The model under review builds one solid part; all positions refer to its coordinate system, in mm. A direction names the side the tool comes from. Round coordinates to 2 decimals unless told otherwise and drop trailing zeros. Loops run counter-clockwise (first coordinate to the right, second up) from the corner with the lowest first, then second, coordinate; pieces in that order, holes last. Notation, with made-up numbers: M 1,-3 L 22,-3 A11 cw 22,2 Z; hole C -24.75,82 d9. An arc over 180 degrees is marked long. Use a Markdown table: item, result. Add a question column.
```python
from build123d import *

# Parameters (mm, degrees)
F2_DEPTH = 381
F0_W     = 914.4
F0_H     = 609.6
F3_DEPTH = 19.05
F4_REACH = 1907.1780931


with BuildPart() as f2:
    # F1 (on Right) → F2 (new body, symmetric)
    with BuildSketch(Plane.YZ):
        Polygon((-197.9734073051, 940.2559094878), (-223.3734073051, 984.25), (-239.8711912472, 974.725), (-204.9461912472, 914.2331255457), (207.4984073051, 1152.3581255457), (197.9734073051, 1168.8559094878), align=None)
    extrude(amount=F2_DEPTH, both=True)



with BuildPart() as f3:
    # F0 (on Top) → F3 (new body)
    with BuildSketch(Plane.XY):
        Rectangle(F0_W, F0_H)
        Polygon((-342.9, -111.5645430735), (-190.5, 152.4), (190.5, 152.4), (342.9, -111.5645430735), (326.4022160579, -121.0895430735), (179.5014773719, 133.35), (-179.5014773719, 133.35), (-326.4022160579, -121.0895430735), align=None, mode=Mode.SUBTRACT)
        Polygon((190.5, 152.4), (-190.5, 152.4), (-342.9, -111.5645430735), (-326.4022160579, -121.0895430735), (-179.5014773719, 133.35), (179.5014773719, 133.35), (326.4022160579, -121.0895430735), (342.9, -111.5645430735), align=None)
    extrude(amount=F3_DEPTH)


with BuildPart() as f2_1:
    add(f2.part)

    add(f3.part)  # F4 merges F3
    f4_end = f2_1.faces().sort_by_distance((0, 1.276108029, 1033.2956255457))[0]
    # F0 (on Top) → F4 (join, up to a face of the model that its end follows)
    with BuildSketch(Plane.XY):
        Polygon((190.5, 152.4), (-190.5, 152.4), (-342.9, -111.5645430735), (-326.4022160579, -121.0895430735), (-179.5014773719, 133.35), (179.5014773719, 133.35), (326.4022160579, -121.0895430735), (342.9, -111.5645430735), align=None)
    f4_long = extrude(amount=F4_REACH, mode=Mode.PRIVATE)
    add(split(f4_long, bisect_by=f4_end, keep=Keep.TOP, mode=Mode.PRIVATE))


solid = f2_1.part
```
(1) To check wall thickness, follow probe 1 along X at (y, z) = (-101, 889.5); probe 2 along Y at (x, z) = (-39.5, 340); probe 3 along X at (y, z) = (-26.5, 463.5). State the ranges of each line that lie inside material, in increasing order.
(2) Consider section C-C, the plane x = 20. Give the boundary of the cut face in (y, z) (3 decimals), then the cut area to 3 significant figures.
(3) Consider section A-A, the plane z = 704.5. Give the boundary of the cut face in (x, y).
(4) Consider section B-B, the plane y = 71.5. Give the boundary of the cut face in (x, z).
(5) For faces 5 (the face through (-381, -34, 1023)), 6 (the face through (267.767, 18.57, 562.088)), 7 (the face through (3, 152.4, 562)), 8 (the face through (-3, 133.35, 557)), 9 (the face through (5.33, -222.65, 944.9)), list the 3-axis set-ups (+Z, -Z, +X, -X, +Y, -Y) from which the entire face can be reached by the end or side of a thin tool; tool diameter is ignored.
(6) Consider section D-D, the plane z = 1056. Give the boundary of the cut face in (x, y).
(7) Draft analysis for pull direction Y (two halves, no side actions). For faces 1 (the face through (381, -34, 1023)), 2 (the face through (5.334, 2.772, 1056.156)), 3 (the face through (-265.63, 22.27, 562.09)), 4 (the face through (5.334, -210.496, 961.945)), state which applies: released by +Y, released by -Y, zero draft, split by the parting line, or undercut.
(8) Insertion check: pin 1 Ø1.5 at (x, y) = (273.5, -224.5) entering from +Z; pin 2 Ø1 at (y, z) = (-76.5, 256.5) entering from +X; pin 3 Ø1 at (y, z) = (128, 698.5) entering from +X; pin 4 Ø6 at (x, y) = (252, 127) entering from -Z. Each pin has a flat end and moves straight along its axis. Give the tip position at first contact, or say it passes through.
Found:
| question | item | result |
|---|---|---|
| 1 | probe 1 | x = -336.8 to -314.8, 314.8 to 336.8 |
| 1 | probe 2 | y = 133.35 to 152.4 |
| 1 | probe 3 | x = -293.79 to -271.79, 271.79 to 293.79 |
| 2 | outline | M -304.8,0 L 304.8,0 L 304.8,19.05 L 152.4,19.05 L 152.4,1120.547 L 207.498,1152.358 L 197.973,1168.856 L -197.973,940.256 L -223.373,984.25 L -239.871,974.725 L -204.946,914.233 L 133.35,1109.549 L 133.35,19.05 L -304.8,19.05 Z |
| 2 | area | 42,500 mm^2 |
| 3 | outline | M -342.9,-111.56 L -326.4,-121.09 L -179.5,133.35 L 179.5,133.35 L 326.4,-121.09 L 342.9,-111.56 L 190.5,152.4 L -190.5,152.4 Z |
| 4 | outline | M -457.2,0 L 457.2,0 L 457.2,19.05 L 237.21,19.05 L 237.21,1073.84 L 381,1073.84 L 381,1095.84 L -381,1095.84 L -381,1073.84 L -237.21,1073.84 L -237.21,19.05 L -457.2,19.05 Z; hole M -215.21,19.05 L 215.21,19.05 L 215.21,1073.84 L -215.21,1073.84 Z |
| 5 | face 5 | +Z, -X, +Y, -Y |
| 5 | face 6 | +X, +Y |
| 5 | face 7 | +X, -X, +Y |
| 5 | face 8 | none |
| 5 | face 9 | +X, -X, -Y |
| 6 | outline | M -381,2.5 L 381,2.5 L 381,40.6 L 255.05,40.6 L 190.5,152.4 L -190.5,152.4 L -255.05,40.6 L -381,40.6 Z; hole M -233.05,40.6 L 233.05,40.6 L 179.5,133.35 L -179.5,133.35 Z |
| 7 | face 1 | zero draft |
| 7 | face 2 | undercut |
| 7 | face 3 | released by +Y |
| 7 | face 4 | undercut |
| 8 | pin 1 | stops at z = 984.03 |
| 8 | pin 2 | stops at x = 322.94 |
| 8 | pin 3 | stops at x = 204.88 |
| 8 | pin 4 | stops at z = 0 |
